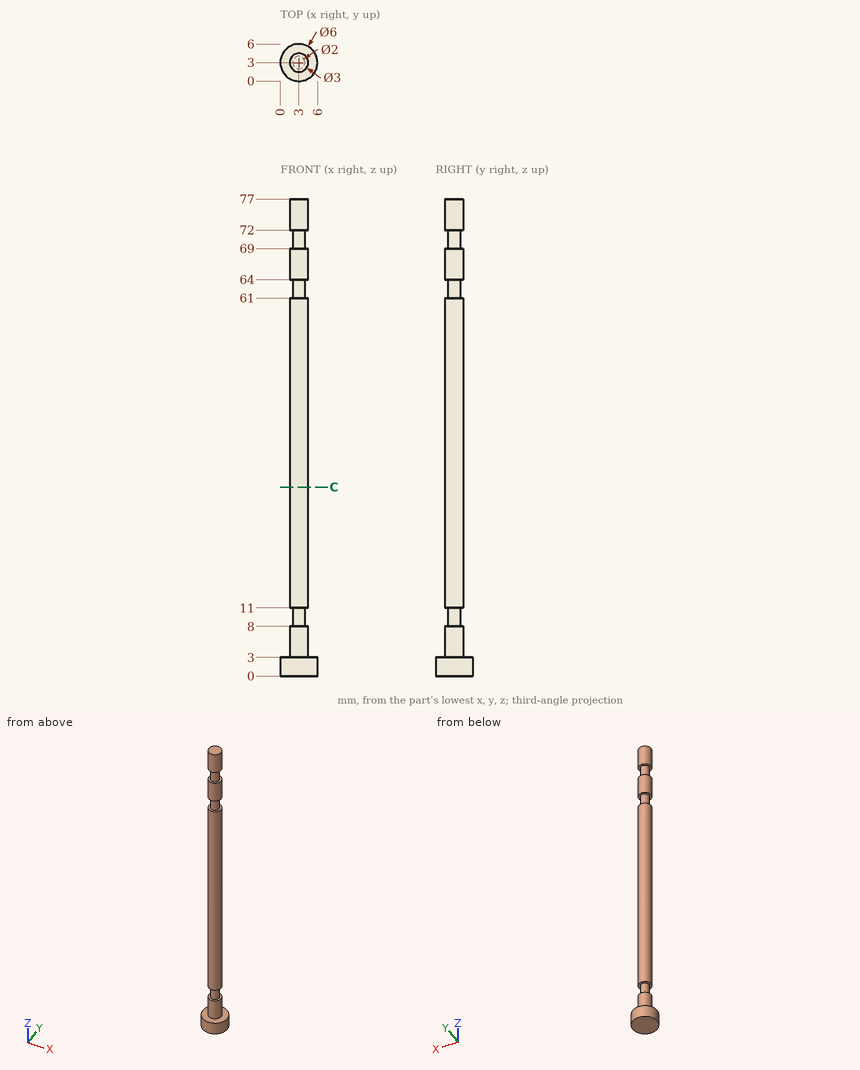
Source: three-view drawing plus pictorial views. Frame: mm from the lowest corner of the part. Give positions to 0.01 mm unless a question says otherwise; leave off trailing zeros. Write each loop counter-clockwise with the first axis right and the second up, starting at its lowest first coordinate (ties: lowest second). Pieces come first, ordered by that corner, then holes. Notation, with made-up numbers: M 48.25,-30 L 74.25,-30 A15 ccw 74.25,-7 Z; hole C -30,66 d11. An arc over 180 degrees is marked long. Use one line per item in the form item = value.
1. First-contact query: P1, Ø3, axis at x = 2.5, y = 5, coming from the +Z side; P2, Ø2, axis at y = 2, z = 56, coming from the -X side; P3, Ø3, axis at x = 5, z = 60, coming from the +Y side. Flat tips, straight axial feed; report the tip coordinate or a pass-through.
Outcome:
P1 = 77
P2 = 1.5
P3 = 4.41
2. Cut plane C-C on z = 30.5. Return loops of the section in (x, y).
Outcome:
outline = C 3,3 d3
3. Ray query, L1, parallel to Z at x = 3.85, y = 3.75; L2, parallel to Z at x = 1.5, y = 1.1; L3, parallel to Y at x = 2.9, z = 71. Return the intervals inside material, ascending.
Outcome:
L1 = 0 to 8, 11 to 61, 64 to 69, 72 to 77
L2 = 0 to 3
L3 = 2.01 to 3.99
